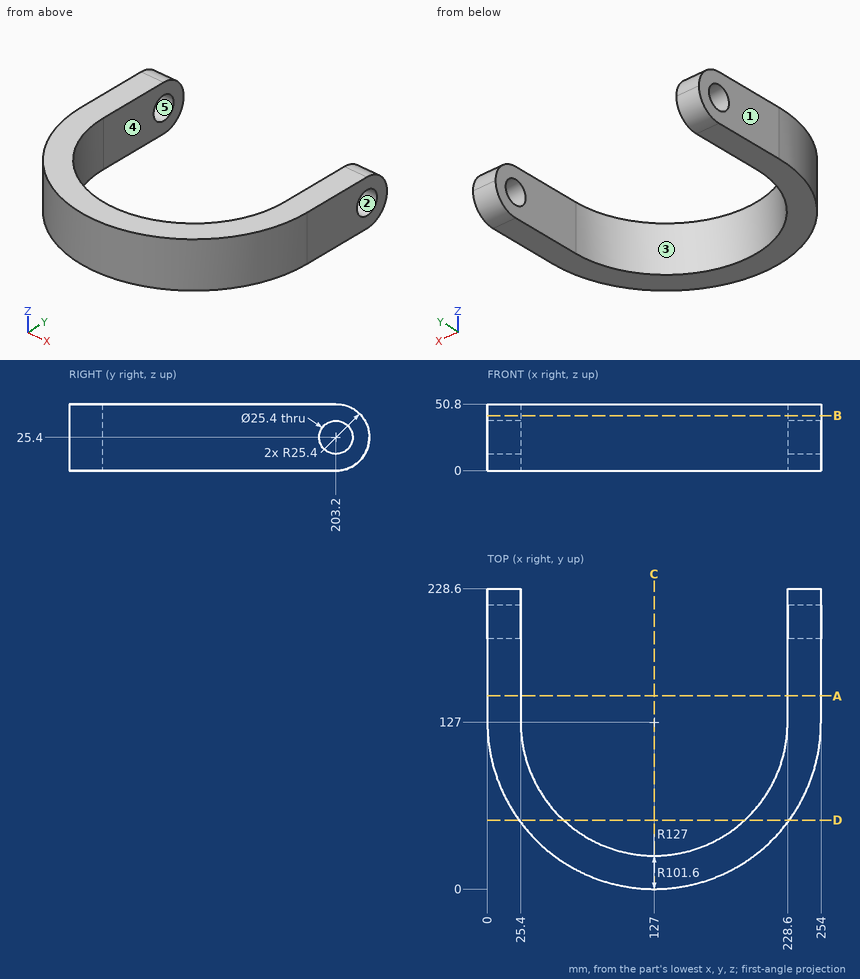
Could you check a few things on this drawing? It's one solid part, dimensions in mm from its lowest x, y, z. A direction names the side the tool comes from. Coordinates: 2 decimals unless noted, no trailing zeros. Write each loop counter-clockwise with the first axis right and the second up, starting at its lowest first coordinate (ties: lowest second). Pieces come first, ordered by that corner, then holes. Notation, with made-up numbers: (9.5, -13.5) - (13.5, -13.5) arc R26 ccw to (13.5, 10.5) - close; hole circle Ø10 at (12.25, -13). An arc over 180 degrees is marked (long way). Use one line per item in the form item = value.
1) Suppose I cut it at A-A, the plane y = 147. Write out the boundary of the cut face in (x, z), plus the area to 3 significant figures.
Solved:
outline = (0, 0) - (25.4, 0) - (25.4, 50.8) - (0, 50.8) - close; (228.6, 0) - (254, 0) - (254, 50.8) - (228.6, 50.8) - close
area = 2,580 mm2
2) Thinking about a two-plate mould opening in Y: for the marked faces 1, 2 and 3, which applies, released by +Y, released by -Y, zero draft, split by the parting line, or undercut?
Solved:
face_1 = zero draft
face_2 = undercut
face_3 = released by +Y
3) On a 3-axis mill with a long thin cutter (end or side, diameter ignored), from which of +Z, -Z, +X, -X, +Y, -Y can I reach the whole of each face in a straight line? I mean the marked faces 4 and 5. Say none if no direction works.
Solved:
face_4 = +Z, -Z, +Y
face_5 = +X, -X
4) Suppose I cut it at D-D, the plane y = 52.5. Write out the boundary of the cut face in (x, z).
Solved:
outline = (24.15, 0) - (57.92, 0) - (57.92, 50.8) - (24.15, 50.8) - close; (196.08, 0) - (229.85, 0) - (229.85, 50.8) - (196.08, 50.8) - close
5) Suppose I cut it at B-B, the plane z = 42. Write out the boundary of the cut face in (x, y) (3 decimals), plus the area to 3 significant figures.
Solved:
outline = (0, 127) arc R127 ccw to (254, 127) - (254, 222.425) - (228.6, 222.425) - (228.6, 127) arc R101.6 cw to (25.4, 127) - (25.4, 222.425) - (0, 222.425) - close
area = 14,000 mm2
6) I'm going to push flat-ended pins straight in: P1, Ø3, axis at x = 90, z = 43.5, coming from the +Y side; P2, Ø15, axis at y = 203.2, z = 25.4, coming from the +X side; P3, Ø8, axis at x = 82.5, z = 41.5, coming from the -Y side; P4, Ø8, axis at x = 98.5, z = 39.5, coming from the +Y side. Where does each tip first touch, or does it pass through?
Solved:
P1 = 32.98
P2 = through
P3 = 6.63
P4 = 30.74
7) I need wall thicknesses on line 1 (X direction, y = 161, z = 23); line 2 (Z direction, x = 7, y = 203.2); line 3 (Y direction, x = 239.5, z = 25.4). Which ranges of each line are inside material? Lowest first, please.
Solved:
line_1 = 0 to 25.4, 228.6 to 254
line_2 = 0 to 12.7, 38.1 to 50.8
line_3 = 68.07 to 190.5, 215.9 to 228.6
8) Suppose I cut it at C-C, the plane x = 127. Write out the boundary of the cut face in (y, z).
Solved:
outline = (0, 0) - (25.4, 0) - (25.4, 50.8) - (0, 50.8) - close
